The model under review builds one solid part; all positions refer to its coordinate system, in mm. A direction names the side the tool comes from. Coordinates: 2 decimals unless noted, no trailing zeros. Loops run counter-clockwise (first coordinate to the right, second up) from the corner with the lowest first, then second, coordinate; pieces in that order, holes last. Notation, with made-up numbers: (27, 33.5) - (85, 33.5) arc R3 cw to (85, 37.5) - close; hole circle Ø4 at (79, 51). An arc over 180 degrees is marked (long way). Answer in a Markdown table with one row per item. Add a question column.
(1) Machinability: for faces 1 (the flat face through (0, 0, 6.35)), 2 (the cylindrical face through (8.61, -4.38, 3.13)), which of the approach directions +Z, -Z, +X, -X, +Y, -Y give a long, thin tool a straight path to every point of the face, cutting with its end or side? Answer none if there is none.
(2) For P1, Ø2.5, axis at x = -21.85, y = 0, coming from the -Z side; P2, Ø2, axis at y = 0.5, z = 5.5, coming from the +X side; P3, Ø1.5, axis at y = -2, z = 3, coming from the +X side; P4, Ø1.5, axis at y = 1, z = 1, coming from the -X side, all flat-tipped, find the tip position at first contact; note any pin that passes through.
(3) We need section B-B on y = 3.5. Write out the cut boundary in (x, z), plus the area to 3 significant figures.
(4) Mouldability with a two-part tool opening along X and no side actions: class faces 3 (the cylindrical face through (-26.613, -0.105, 3.131)), 4 (the cylindrical face through (14.24, -4.4, 3.13)), 5 (the flat face through (0, 0, 0)) as +X half, -X half, draft (parallel to the pull), parting line (faces both ways), or undercut.
(5) We need section A-A on z = 4.5. Give the number of separate pieces and of enclosed holes in the cut face, plus the area to 3 significant figures.
(6) For line 1 along X through (y, z) = (-0.25, 5.5); line 2 along X through (y, z) = (-0.5, 1); line 3 along X through (y, z) = (-4, 5), list the stretches that pass through material, from the lowest coordinate up.
(7) We need section C-C on x = 11.5. Write out the cut boundary in (y, z).
from build123d import *

# Parameters (mm, degrees)
SKETCH1_R           = 1.65
BOSS_EXTRUDE1_DEPTH = 6.35
CUT_EXTRUDE3_DEPTH  = 28.772450308


with BuildPart() as part:
    # Sketch1 → Boss-Extrude1 (new body)
    with BuildSketch(Plane.XY):
        with BuildLine():
            Line((-21.851501763, 4.7625), (21.851501763, 4.7625))
            ThreePointArc((21.851501763, 4.7625), (26.614001763, 0), (21.851501763, -4.7625))
            Line((21.851501763, -4.7625), (-21.851501763, -4.7625))
            ThreePointArc((-21.851501763, -4.7625), (-26.614001763, 0), (-21.851501763, 4.7625))
        make_face()
        with Locations((21.851501763, 0)):
            Circle(SKETCH1_R, mode=Mode.SUBTRACT)
        with Locations((-21.851501763, 0)):
            Circle(SKETCH1_R, mode=Mode.SUBTRACT)
    extrude(amount=BOSS_EXTRUDE1_DEPTH)

    # Sketch4 → Cut-Extrude3 (cut, through all)
    with BuildSketch(Plane(origin=(0, 0, 0), x_dir=(-1, 0, 0), z_dir=(0, 0, -1))):
        with BuildLine():
            Line((-8.969452091, 0), (-8.969452091, -3.4925))
            ThreePointArc((-8.969452091, -3.4925), (-8.597477703, -4.390525612), (-7.699452091, -4.7625))
            Line((-7.699452091, -4.7625), (-15.126952091, -4.7625))
            ThreePointArc((-15.126952091, -4.7625), (-14.228926479, -4.390525612), (-13.856952091, -3.4925))
            Line((-13.856952091, -3.4925), (-13.856952091, 0))
            ThreePointArc((-13.856952091, 0), (-11.413202091, 2.44375), (-8.969452091, 0))
        make_face()
    extrude(amount=-CUT_EXTRUDE3_DEPTH, mode=Mode.SUBTRACT)


solid = part.part
Outcome:
| question | item | result |
|---|---|---|
| 1 | face 1 | +Z, +X, -X, +Y, -Y |
| 1 | face 2 | +Z, -Z, -Y |
| 2 | P1 | through |
| 2 | P2 | x = 26.61 |
| 2 | P3 | x = 26.45 |
| 2 | P4 | x = -26.61 |
| 3 | outline | (-25.08, 0) - (25.08, 0) - (25.08, 6.35) - (-25.08, 6.35) - close |
| 3 | area | 319 mm² |
| 4 | face 3 | -X half |
| 4 | face 4 | undercut |
| 4 | face 5 | draft |
| 5 | separate pieces | 1 |
| 5 | enclosed holes | 2 |
| 5 | area | 437 mm² |
| 6 | line 1 | -26.61 to -23.48, -20.22 to 8.97, 13.86 to 20.22, 23.48 to 26.61 |
| 6 | line 2 | -26.59 to -23.42, -20.28 to 8.97, 13.86 to 20.28, 23.42 to 26.59 |
| 6 | line 3 | -24.44 to 8.86, 13.96 to 24.44 |
| 7 | outline | (2.44, 0) - (4.76, 0) - (4.76, 6.35) - (2.44, 6.35) - close |
